Design review of the part built by this model. Coordinates are the model's own, in mm. A direction names the side the tool comes from. Coordinates: 2 decimals unless noted, no trailing zeros. Write each loop counter-clockwise with the first axis right and the second up, starting at its lowest first coordinate (ties: lowest second). Pieces come first, ordered by that corner, then holes. Notation, with made-up numbers: (-1.5, -36.75) - (54.5, -36.75) arc R32 cw to (54.5, -1.75) - close; hole circle Ø1 at (-39.5, 66.5). An arc over 180 degrees is marked (long way). Use a Markdown table: item, result.
from build123d import *

# Parameters (mm, degrees)
SKETCH1_W           = 76.2
SKETCH1_H           = 25.4
BOSS_EXTRUDE1_DEPTH = 7.62
SKETCH2_R           = 0.863384433
CUT_EXTRUDE1_DEPTH  = 6.35
CHAMFER1_SIZE       = 0.508
SKETCH3_W           = 12.7
SKETCH3_H           = 19.05
BOSS_EXTRUDE2_DEPTH = 7.62


with BuildPart() as part:
    # Sketch1 → Boss-Extrude1 (new body)
    with BuildSketch(Plane.XY):
        with Locations((38.1, 12.7)):
            Rectangle(SKETCH1_W, SKETCH1_H)
    extrude(amount=BOSS_EXTRUDE1_DEPTH)

    # Sketch2 → Cut-Extrude1 (cut)
    with BuildSketch(Plane(origin=(0, 0, 0), x_dir=(-1, 0, 0), z_dir=(0, 0, -1))):
        with Locations((-25.4, 12.7)):
            Circle(SKETCH2_R)
        Polygon((-28.388596798, 21.04725), (-32.311403202, 21.04725), (-34.272806404, 17.65), (-32.311403202, 14.25275), (-28.388596798, 14.25275), (-26.427193596, 17.65), align=None)
        Polygon((-18.488596798, 21.04725), (-22.411403202, 21.04725), (-24.372806404, 17.65), (-22.411403202, 14.25275), (-18.488596798, 14.25275), (-16.527193596, 17.65), align=None)
        Polygon((-18.488596798, 11.14725), (-22.411403202, 11.14725), (-24.372806404, 7.75), (-22.411403202, 4.35275), (-18.488596798, 4.35275), (-16.527193596, 7.75), align=None)
        Polygon((-28.388596798, 11.14725), (-32.311403202, 11.14725), (-34.272806404, 7.75), (-32.311403202, 4.35275), (-28.388596798, 4.35275), (-26.427193596, 7.75), align=None)
    extrude(amount=-CUT_EXTRUDE1_DEPTH, mode=Mode.SUBTRACT)

    # Chamfer1
    chamfer1_edges = [part.edges().sort_by_distance(p)[0] for p in [
        (27.407895197, 9.448625, 0),
        (30.35, 11.14725, 0),
        (33.292104803, 9.448625, 0),
        (33.292104803, 6.051375, 0),
        (30.35, 4.35275, 0),
        (27.407895197, 6.051375, 0),
        (17.507895197, 9.448625, 0),
        (20.45, 11.14725, 0),
        (23.392104803, 9.448625, 0),
        (23.392104803, 6.051375, 0),
        (20.45, 4.35275, 0),
        (17.507895197, 6.051375, 0),
        (17.507895197, 19.348625, 0),
        (20.45, 21.04725, 0),
        (23.392104803, 19.348625, 0),
        (23.392104803, 15.951375, 0),
        (20.45, 14.25275, 0),
        (17.507895197, 15.951375, 0),
        (27.407895197, 19.348625, 0),
        (30.35, 21.04725, 0),
        (33.292104803, 19.348625, 0),
        (33.292104803, 15.951375, 0),
        (30.35, 14.25275, 0),
        (27.407895197, 15.951375, 0),
    ]]
    chamfer(chamfer1_edges, length=CHAMFER1_SIZE)

    # Sketch3 → Boss-Extrude2 (add)
    with BuildSketch(Plane(origin=(0, 0, 0), x_dir=(-1, 0, 0), z_dir=(0, 0, -1))):
        with Locations((-25.4, -9.525)):
            Rectangle(SKETCH3_W, SKETCH3_H)
        with Locations((-25.4, 34.925)):
            Rectangle(SKETCH3_W, SKETCH3_H)
    extrude(amount=-BOSS_EXTRUDE2_DEPTH)


solid = part.part
(1) Machinability: for faces 1 (the flat face through (19.05, -10, 4)), 2 (the flat face through (31.75, -10, 4)), 3 (the flat face through (23.6, 6, 0.3)), 4 (the flat face through (38, 13, 0)), which of the approach directions +Z, -Z, +X, -X, +Y, -Y give a long, thin tool a straight path to every point of the face, cutting with its end or side? Answer none if there is none.
Determined:
| item | result |
|---|---|
| face 1 | +Z, -Z, -X, -Y |
| face 2 | +Z, -Z, +X, -Y |
| face 3 | -Z |
| face 4 | -Z, +X, -X, +Y, -Y |
(2) Take a section at B-B on x = 71.5. Write out the cut boundary in (y, z), and give its area (3 significant figures).
Determined:
| item | result |
|---|---|
| outline | (0, 0) - (25.4, 0) - (25.4, 7.62) - (0, 7.62) - close |
| area | 194 mm2 |
(3) Draft analysis for pull direction Y (two halves, no side actions). For faces 5 (the flat face through (20, 14.253, 3)), 6 (the flat face through (31.75, 35, 4)), 7 (the flat face through (25, 44.45, 4)), state which applies: +Y half, -Y half, draft (parallel to the pull), parting line (faces both ways), or undercut.
Determined:
| item | result |
|---|---|
| face 5 | undercut |
| face 6 | draft |
| face 7 | +Y half |
(4) Take a section at D-D on y = -13.5. Write out the cut boundary in (x, z), and give its area (3 significant figures).
Determined:
| item | result |
|---|---|
| outline | (19.05, 0) - (31.75, 0) - (31.75, 7.62) - (19.05, 7.62) - close |
| area | 96.8 mm2 |
(5) Take a section at A-A on y = 12.7. Write out the cut boundary in (x, z), and give its area (3 significant figures).
Determined:
| item | result |
|---|---|
| outline | (0, 0) - (24.54, 0) - (24.54, 6.35) - (26.26, 6.35) - (26.26, 0) - (76.2, 0) - (76.2, 7.62) - (0, 7.62) - close |
| area | 570 mm2 |
(6) For pin 1 (4 mm diameter, centred on y = 33, z = 4, fed in from +X); pin 2 (12 mm diameter, centred on x = 17.5, y = -3, fed in from -Z), all flat-tipped, find the tip position at first contact; note any pin that passes through.
Determined:
| item | result |
|---|---|
| pin 1 | x = 31.75 |
| pin 2 | z = 0 |
(7) Take a section at C-C on z = 4. State how many separate pieces and enclosed holes the cut face has, and give its area (3 significant figures).
Determined:
| item | result |
|---|---|
| separate pieces | 1 |
| enclosed holes | 5 |
| area | 2,260 mm2 |
(8) For L1, parallel to Y at x = 21, z = 4.25; L2, parallel to Y at x = 32, z = 3; L3, parallel to Y at x = 25.4, z = 1.5, list the stretches that pass through material, from the lowest coordinate up. Write a range as from..to.
Determined:
| item | result |
|---|---|
| L1 | -19.05..4.35, 11.15..14.25, 21.05..44.45 |
| L2 | 0..4.35, 11.15..14.25, 21.05..25.4 |
| L3 | -19.05..11.84, 13.56..44.45 |
